Autodesk Inventor part; units mm, degrees
ref_plane "Work Plane2" through (-3.048, 41.148, 101.6) normal (0, 0.2588, 0.9659) x (-1, 0, 0)
ref_plane "YZ Plane" through (0, 0, 0) normal (1, 0, 0) x (0, 1, 0)
ref_plane "XZ Plane" through (0, 0, 0) normal (0, 1, 0) x (-1, 0, 0)
sketch "Sketch1" plane through (0, 0, 0) normal (0, 0, 1) x (1, 0, 0)
  line L0 (0, 0) -> (88.9, 0)
  line L1 (88.9, 0) -> (88.9, 38.1)
  line L2 (88.9, 38.1) -> (0, 38.1)
  line L3 (0, 38.1) -> (0, 0)
  line L4 (-3.048, 41.148) -> (91.948, 41.148)
  line L5 (91.948, 41.148) -> (91.948, -3.048)
  line L6 (91.948, -3.048) -> (-3.048, -3.048)
  line L7 (-3.048, -3.048) -> (-3.048, 41.148)
  dimension "d0" = 88.9
  dimension "d1" = 38.1
  dimension "d2" = 3.048
extrude "Extrusion1" add sketch "Sketch1" along normal blind 101.6
ref_plane "Work Plane2" through (-3.048, 41.148, 101.6) normal (0, 0.2588, 0.9659) x (-1, 0, 0)
sketch "Sketch3" plane through (-3.048, 41.148, 101.6) normal (0, 0.2588, 0.9659) x (-1, 0, 0)
  line L0 (-130.175, -76.2) -> (53.975, -76.2)
  line L1 (53.975, -76.2) -> (53.975, 57.15)
  line L2 (53.975, 57.15) -> (-130.175, 57.15)
  line L3 (-130.175, 57.15) -> (-130.175, -76.2)
  point P0 (-3.048, 13.4499)
extrude "Extrusion3" cut sketch "Sketch3" against normal blind 12.7
properties part number "endHoriz" material "Steel, Galvanized"
Can you work these out from the model? Positions are in its coordinate system, mm. A direction names the side the tool comes from. Coordinates: 2 decimals unless noted, no trailing zeros. Order: outer loops, then holes, each group sorted by start corner. A loop starts at its lowest first (then second) coordinate and runs counter-clockwise, first axis right, second up. Notation, with made-up numbers: M 23,-31.75 L 60,-31.75 A13 cw 60,-15.75 Z; hole C 58.25,-31.75 d10. An arc over 180 degrees is marked long. Answer as CSV lines item,"result".
(1) Suppose I cut it at C-C on y = 33. Please give me the cut outline in (x, z), plus the area to 4 significant figures.
Geometry check:
outline,"M -3.05,0 L 0,0 L 0,90.63 L -3.05,90.63 Z; M 88.9,0 L 91.95,0 L 91.95,90.63 L 88.9,90.63 Z"
area,"552.5 mm^2"
(2) Suppose I cut it at D-D on z = 93.5. Please give me the cut outline in (x, y).
Geometry check:
outline,"M -3.05,-3.05 L 91.95,-3.05 L 91.95,22.3 L 88.9,22.3 L 88.9,0 L 0,0 L 0,22.3 L -3.05,22.3 Z"
(3) Please list where these lines run through material, in increasing order: L1, parallel to Y at x = 23, z = 55; L2, parallel to X at y = 1.5, z = 56.5; L3, parallel to Y at x = 28, z = 93.
Geometry check:
L1,"-3.05 to 0, 38.1 to 41.15"
L2,"-3.05 to 0, 88.9 to 91.95"
L3,"-3.05 to 0"
(4) Suppose I cut it at A-A on z = 57. Please give me the cut outline in (x, y), plus the area to 3 significant figures.
Geometry check:
outline,"M -3.05,-3.05 L 91.95,-3.05 L 91.95,41.15 L -3.05,41.15 Z; hole M 0,0 L 88.9,0 L 88.9,38.1 L 0,38.1 Z"
area,"811 mm^2"
(5) If we mould it in two halves opening along Y, with no side actions, what happens to faces 1 (the flat face through (45, -3.048, 49)), 2 (the flat face through (44, 41.148, 44)), 3 (the flat face through (45, 38.1, 44)), 4 (the flat face through (44, 0, 49))? For each: released by +Y, released by -Y, zero draft, split by the parting line, or undercut.
Geometry check:
face 1,"released by -Y"
face 2,"released by +Y"
face 3,"undercut"
face 4,"undercut"
(6) Suppose I cut it at B-B on x = 7. Please give me the cut outline in (y, z).
Geometry check:
outline,"M -3.05,0 L 0,0 L 0,99.48 L -3.05,100.29 Z; M 38.1,0 L 41.15,0 L 41.15,88.45 L 38.1,89.27 Z"
(7) On a 3-axis mill with a long thin cutter (end or side, diameter ignored), from which of +Z, -Z, +X, -X, +Y, -Y can I reach the whole of each face in a straight line? I mean faces 5 (the flat face through (0, 19, 49)), 6 (the flat face through (48.19, 38.59, 89.135)). Say none if no direction works.
Geometry check:
face 5,"+Z, -Z"
face 6,"+Z, +X, -X, +Y"
(8) I'm going to push a flat-ended pin straight in: pin 1 (6 mm diameter, centred on x = 52.5, y = 35.5, fed in from +Z). Where does the tip first touch, or does it pass through?
Geometry check:
pin 1,"z = 89.27"
